Study the drawing (mm; zero at the part's minimum x, y, z) and answer. Round coordinates to 2 decimals unless told otherwise and drop trailing zeros. Loops run counter-clockwise (first coordinate to the right, second up) from the corner with the lowest first, then second, coordinate; pieces in that order, holes last. Notation, with made-up numbers: M 56.25,71 L 106.25,71 A33 ccw 106.25,102 Z; hole C 33.5,51 d10. An arc over 180 degrees is marked long. Write each question's results on one line, items separated by ' | '.
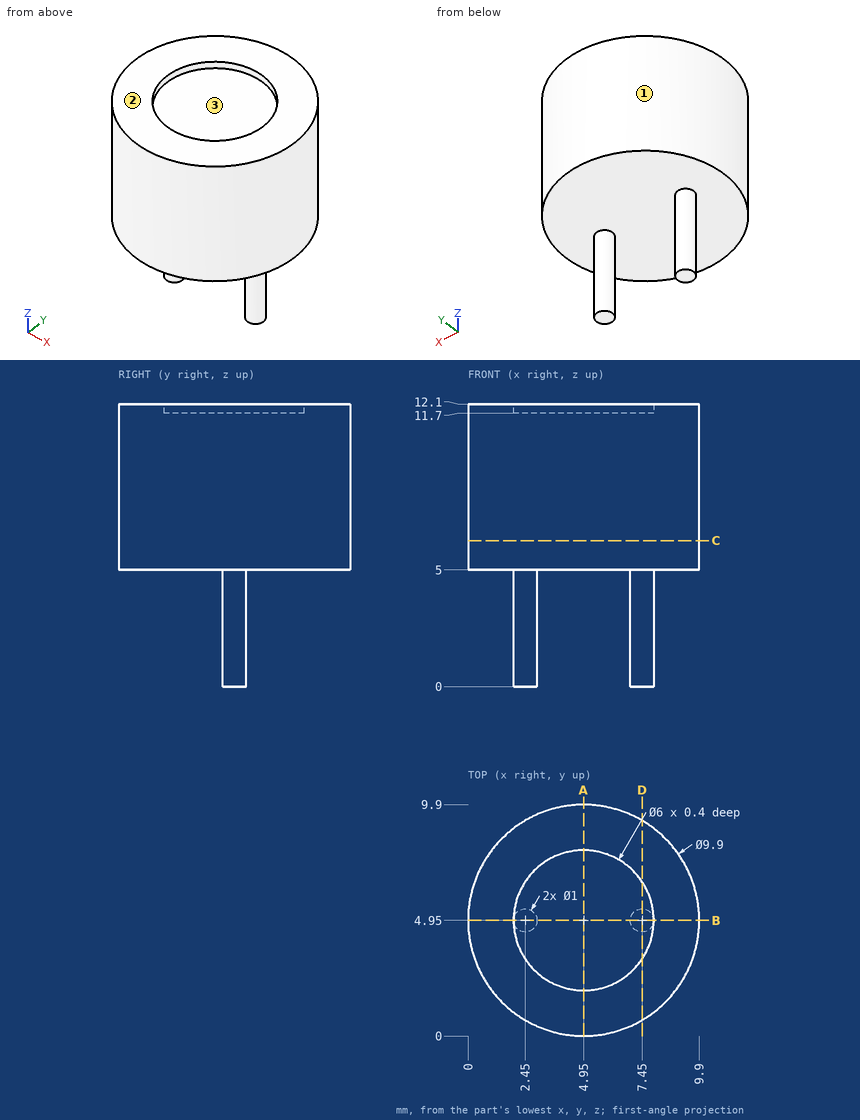
Item 1: The mould has two halves that part along Y. Classify the marked faces 1, 2 and 3: pulls with the +Y half, pulls with the -Y half, needs draft (parallel to the pull), parting line crosses it, or undercut.
Outcome:
face 1: parting line crosses it | face 2: needs draft | face 3: undercut
Item 2: The part is cut by section C-C (z = 6.25). Determine the outline of the cut face in (x, y).
Outcome:
outline: C 4.95,4.95 d9.9
Item 3: Straight lines are drawn through the part: line 1 (Y direction, x = 4.95, z = 12.05); line 2 (Z direction, x = 1.5, y = 3.75); line 3 (Z direction, x = 5.5, y = 5.75). For each, find the intervals that lie inside material, in ascending order.
Outcome:
line 1: y = 0 to 1.95, 7.95 to 9.9 | line 2: z = 5 to 12.1 | line 3: z = 5 to 11.7
Item 4: The part is cut by section B-B (y = 4.95). Determine the outline of the cut face in (x, z).
Outcome:
outline: M 0,5 L 1.95,5 L 1.95,0 L 2.95,0 L 2.95,5 L 6.95,5 L 6.95,0 L 7.95,0 L 7.95,5 L 9.9,5 L 9.9,12.1 L 7.95,12.1 L 7.95,11.7 L 1.95,11.7 L 1.95,12.1 L 0,12.1 Z
Item 5: The part is cut by section D-D (x = 7.45). Determine the outline of the cut face in (y, z).
Outcome:
outline: M 0.68,5 L 4.45,5 L 4.45,0 L 5.45,0 L 5.45,5 L 9.22,5 L 9.22,12.1 L 6.61,12.1 L 6.61,11.7 L 3.29,11.7 L 3.29,12.1 L 0.68,12.1 Z
Item 6: The part is cut by section A-A (x = 4.95). Determine the outline of the cut face in (y, z).
Outcome:
outline: M 0,5 L 9.9,5 L 9.9,12.1 L 7.95,12.1 L 7.95,11.7 L 1.95,11.7 L 1.95,12.1 L 0,12.1 Z
Item 7: Flat-ended cylindrical pins translate along their axes: pin 1 (4 mm diameter, centred on x = 6, y = 6, fed in from -Z); pin 2 (2 mm diameter, centred on x = 5, y = 2.5, fed in from -Z); pin 3 (3 mm diameter, centred on y = 6, z = 3, fed in from -X). Find the tip coordinate at first contact, or state that the pin passes through.
Outcome:
pin 1: stops at z = 0 | pin 2: stops at z = 5 | pin 3: stops at x = 1.95
